Verification items for the finished model (mm, model axes). Round coordinates to 2 decimals unless told otherwise and drop trailing zeros. Write each loop counter-clockwise with the first axis right and the second up, starting at its lowest first coordinate (ties: lowest second). Pieces come first, ordered by that corner, then holes. Notation, with made-up numbers: (7, -25.75) - (12, -25.75) arc R35 cw to (12, 13.25) - close; hole circle Ø1 at (-32, 11). An arc over 180 degrees is marked (long way). Answer as a JSON object with one key per item and string values.
```python
from build123d import *

# Parameters (mm, degrees)
F2_T = -8


# Not quite as in the source:
# - a fillet or chamfer that OpenCascade refuses, or shapes differently, is made with other operations: its cross-section is extruded or revolved along the edge and cut away or added


with BuildPart() as f1:
    # F0 (on Front) → F1 (revolve)
    with BuildSketch(Plane.XZ):
        Polygon((-120, 0), (0, 0), (0, 393.8273733503), (-190, 393.8273733503), align=None)
    revolve(axis=Axis((0, 0, 196.9136866752), (0, 0, -1)))

    # F2
    f2_openings = [f1.faces().sort_by_distance(p)[0] for p in [
        (0, 0, 393.827373),
    ]]
    offset(amount=F2_T, openings=f2_openings)

    # F3: fillet of radius 10 on 1 edges, made by hand

    # F3_s1 → F3_t2 (revolve, cut)
    with BuildSketch(Plane.XZ):
        with BuildLine():
            ThreePointArc((-190, 393.8273733503), (-183.7348569365, 391.4131139305), (-180.408809713, 385.5806122358))
            Line((-180.408809713, 385.5806122358), (-181.8746125421, 393.8273733503))
            Line((-181.8746125421, 393.8273733503), (-190, 393.8273733503))
        make_face()
    revolve(axis=Axis((0, 0, 393.8273733503), (0, 0, -1)), mode=Mode.SUBTRACT)


solid = f1.part
```
Q1. Release check for a two-part mould opening along X. For faces 1 (the conical face through (116.442, -89.284, 150.398)), 2 (the conical face through (30.12, -135.62, 152.19)), 3 (the flat face through (2, 2, 0)) record: released by +X, released by -X, zero draft, split by the parting line, or undercut.
Geometry check:
{"face 1": "split by the parting line", "face 2": "undercut", "face 3": "zero draft"}
Q2. Gauge pin test, flat ends, axial feed: P1, Ø10, axis at x = -94.5, y = 43.5, coming from the +Z side; P2, Ø1, axis at x = -77.5, z = 134, coming from the -Y side; P3, Ø12, axis at x = 7.5, z = 92.5, coming from the +Y side. Record the tip position at first contact, or that the pin passes through.
Geometry check:
{"P1": "stops at z = 8", "P2": "stops at y = -121.49", "P3": "stops at y = 137.34"}
Q3. Section check D-D, the plane z = 53. Record the cut outline in (x, y).
Geometry check:
{"outline": "circle Ø258.84 at (0, 0); hole circle Ø242.59 at (0, 0)"}
Q4. Material ranges on line 1 along Z through (x, y) = (57, -91.5); line 2 along Y through (x, z) = (-54, 146.5); line 3 along Y through (x, z) = (85.5, 326.5), recorded low to high. Write a range as [from, to].
Geometry check:
{"line 1": "z = [0, 8]", "line 2": "y = [-135.69, -126.9], [126.9, 135.69]", "line 3": "y = [-156.16, -146.83], [146.83, 156.16]"}
Q5. Section check C-C, the plane z = 268. Record the cut outline in (x, y), then the cut area to 3 significant figures.
Geometry check:
{"outline": "circle Ø335.27 at (0, 0); hole circle Ø319.02 at (0, 0)", "area": "8,350 mm2"}
Q6. Section check A-A, the plane x = 0. Record the cut outline in (y, z), then the cut area to 3 significant figures.
Geometry check:
{"outline": "(-190, 393.83) - (-120, 0) - (120, 0) - (190, 393.83) arc R10 ccw to (180.41, 385.58) - (113.3, 8) - (-113.3, 8) - (-180.41, 385.58) arc R10 ccw to start", "area": "8,170 mm2"}
